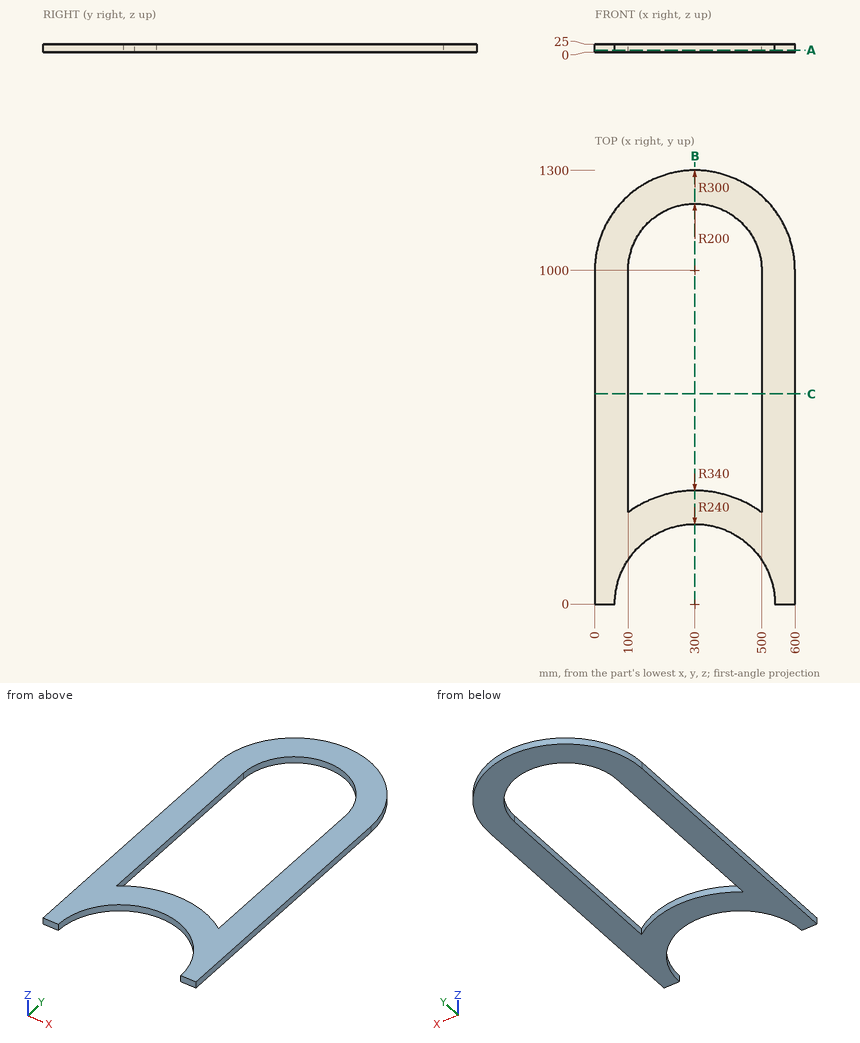
Answer from the drawing. Dimensions are ordinates in mm from the lowest x, y and z of the part. Coordinates: 2 decimals unless noted, no trailing zeros. Order: outer loops, then holes, each group sorted by start corner. A loop starts at its lowest first (then second) coordinate and runs counter-clockwise, first axis right, second up. Notation, with made-up numbers: (-29.5, 60) - (2.5, 60) arc R23 cw to (2.5, 76) - close; hole circle Ø5 at (12.5, 31.5). An arc over 180 degrees is marked (long way). Answer as a JSON object with one key per item and string values. Group by question number.
Item 1: Section B-B (x = 300) is taken. Give the vertices of the cut face in (y, z).
Item 2: Flat-ended cylindrical pins translate along their axes: P1, Ø10, axis at x = 121, z = 4, coming from the -Y side; P2, Ø4, axis at x = 256, z = 3, coming from the -Y side; P3, Ø1, axis at x = 358, z = 17.5, coming from the -Y side. Find the tip coordinate at first contact, or state that the pin passes through.
Item 3: Consider probe 1 along X at (y, z) = (938, 15.75); probe 2 along X at (y, z) = (278.5, 16.5); probe 3 along Y at (x, z) = (308, 14.5). Determine where each line is inside the solid, lowest interval first. Write a range as from..to.
Item 4: Section A-A (z = 6.5) is taken. Give the vertices of the cut face in (x, y).
Item 5: Section C-C (y = 630) is taken. Give the vertices of the cut face in (x, z).
Results are:
{
 "1": {"outline": "(240, 0) - (340, 0) - (340, 25) - (240, 25) - close; (1200, 0) - (1300, 0) - (1300, 25) - (1200, 25) - close"},
 "2": {"P1": "stops at y = 154.09", "P2": "stops at y = 235.55", "P3": "stops at y = 232.76"},
 "3": {"probe 1": "x = 0..100, 500..600", "probe 2": "x = 0..100, 104.97..495.03, 500..600", "probe 3": "y = 239.87..339.91, 1199.84..1299.89"},
 "4": {"outline": "(0, 0) - (60, 0) arc R240 cw to (540, 0) - (600, 0) - (600, 1000) arc R300 ccw to (0, 1000) - close; hole (100, 274.95) arc R340 cw to (500, 274.95) - (500, 1000) arc R200 ccw to (100, 1000) - close"},
 "5": {"outline": "(0, 0) - (100, 0) - (100, 25) - (0, 25) - close; (500, 0) - (600, 0) - (600, 25) - (500, 25) - close"}
}
